CAD build for the part. Positions are in the model's coordinates, mm. Round coordinates to 2 decimals unless told otherwise and drop trailing zeros. Write each loop counter-clockwise with the first axis right and the second up, starting at its lowest first coordinate (ties: lowest second). Pieces come first, ordered by that corner, then holes. Notation, with made-up numbers: (50.5, -12.5) -> (56.5, -12.5) arc R33 ccw to (56.5, 19.5) -> close; hole circle Ø4 at (-40, 4). An arc over 180 degrees is marked (long way). Put each result on its own line as item: value. Start each with the question number.
1. Saw through at A-A on x = -671. List the corners of the cut face in (y, z).
2. Flat gauge pin, fed straight in: P1, Ø1, axis at x = -458.5, z = -8, coming from the -Y side. Where does the tip first touch, or does it go through?
3. Saw through at B-B on z = -10.75. List the corners of the cut face in (x, y).
4. Drill centre lines: line 1 (Y direction, x = -824.5, z = -5); line 2 (Y direction, x = 81, z = -14.75). Where is each one in solid material? Low to high. Write a range as from..to.
from build123d import *

# Parameters (mm, degrees)
SKETCH_1_W             = 2190
SKETCH_1_H             = 184
SM_BASE_FLANGE_1_DEPTH = 18
CUT_EXTRUDE_1_DEPTH    = 2193.005474446


# Sheet-metal steps are written as plain solids
with BuildPart() as part:
    # Sketch 1 → 基体-法兰1 (new body)
    with BuildSketch(Plane.XY):
        Rectangle(SKETCH_1_W, SKETCH_1_H)
    extrude(amount=-SM_BASE_FLANGE_1_DEPTH)

    # 草图6 → 切除-拉伸1 (cut, through all)
    with BuildSketch(Plane.ZY.offset(1095)):
        Polygon((-18, 92), (-18, 80.796679389), (-2, 92), align=None)
        Polygon((-18, -92), (-18, -80.796679389), (-2, -92), align=None)
    extrude(amount=-CUT_EXTRUDE_1_DEPTH, mode=Mode.SUBTRACT)


solid = part.part
Return value:
1. outline: (-92, -2) -> (-80.8, -18) -> (80.8, -18) -> (92, -2) -> (92, 0) -> (-92, 0) -> close
2. P1: stops at y = -88.15
3. outline: (-1095, -85.87) -> (1095, -85.87) -> (1095, 85.87) -> (-1095, 85.87) -> close
4. line 1: y = -89.9..89.9
4. line 2: y = -83.07..83.07
